from build123d import *

# Parameters (mm, degrees)
SKETCH2_W          = 125
SKETCH2_H          = 77.2
BASE_FLANGE1_DEPTH = 2
SKETCH2_3_W        = 3
SKETCH2_3_H        = 1.5
CUT_EXTRUDE1_DEPTH = 2
EDGE_FLANGE1_DEPTH = 50
SKETCH2_4_R        = 5
CUT_EXTRUDE2_DEPTH = 2
SKETCH12_R         = 5.5
CUT_EXTRUDE3_DEPTH = 2
FILLET1_R          = 3


# Sheet-metal steps are written as plain solids
with BuildPart() as part:
    # Sketch2 → Base-Flange1 (new body)
    with BuildSketch(Plane.XY):
        Rectangle(SKETCH2_W, SKETCH2_H)
    extrude(amount=-BASE_FLANGE1_DEPTH)

    # Sketch2<3> → Cut-Extrude1 (cut)
    with BuildSketch(Plane.XY):
        with Locations((-11, -37.85)):
            Rectangle(SKETCH2_3_W, SKETCH2_3_H)
    extrude(amount=-CUT_EXTRUDE1_DEPTH, mode=Mode.SUBTRACT)

    # Edge-Flange1 section (across the edge) → Edge-Flange1 (add)
    with BuildSketch(Plane(origin=(-62.5, -43.6, 0), x_dir=(0, 1, 0), z_dir=(1, 0, 0))):
        with BuildLine():
            Line((0, 0.7366), (0, 64.925))
            Line((0, 64.925), (2, 64.925))
            Line((2, 64.925), (2, 0.7366))
            ThreePointArc((2, 0.7366), (2.215745145, 0.215745145), (2.7366, 0))
            Line((2.7366, 0), (5, 0))
            Line((5, 0), (5, -2))
            Line((5, -2), (2.7366, -2))
            ThreePointArc((2.7366, -2), (0.801531583, -1.198468417), (0, 0.7366))
        make_face()
    extrude(amount=EDGE_FLANGE1_DEPTH)

    # Sketch2<4> → Cut-Extrude2 (cut)
    with BuildSketch(Plane.XY):
        with Locations((12.5, -11.4)):
            Circle(SKETCH2_4_R)
    extrude(amount=-CUT_EXTRUDE2_DEPTH, mode=Mode.SUBTRACT)

    # Sketch12 → Cut-Extrude3 (cut)
    with BuildSketch(Plane.XZ.offset(43.6)):
        with Locations(Location((-37.5, 39.925, 0), (0, 0, 270))):
            Circle(SKETCH12_R)
    extrude(amount=-CUT_EXTRUDE3_DEPTH, mode=Mode.SUBTRACT)

    # Fillet1
    fillet1_edges = [part.edges().sort_by_distance(p)[0] for p in [
        (-62.5, -42.6, 64.925),
        (-12.5, -42.6, 64.925),
        (62.5, 38.6, -1),
        (62.5, -38.6, -1),
        (-62.5, 38.6, -1),
    ]]
    fillet(fillet1_edges, radius=FILLET1_R)


solid = part.part
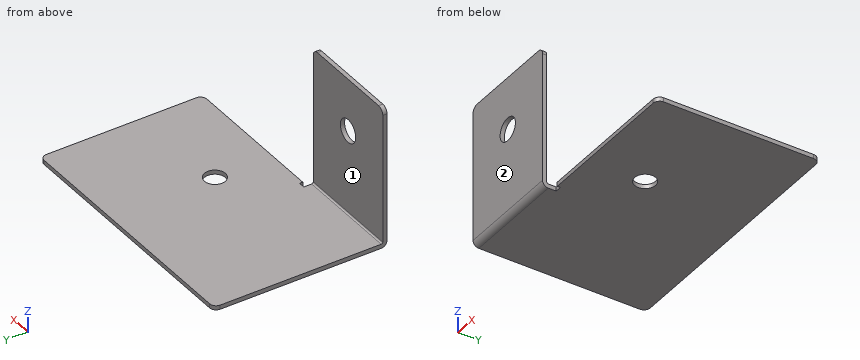
Check sheet for the modelled part. Datum: model origin and axes. Units: mm. Face numbers are marked on the shaded views. A direction names the side the tool comes from. Give positions to 0.01 mm unless a question says otherwise; leave off trailing zeros. Write each loop counter-clockwise with the first axis right and the second up, starting at its lowest first coordinate (ties: lowest second). Pieces come first, ordered by that corner, then holes. Notation, with made-up numbers: (25.25, 52.25) -> (34.25, 52.25) arc R11 cw to (34.25, 67.25) -> close; hole circle Ø7 at (6.5, 81.25). An arc over 180 degrees is marked (long way). Write item = value, one per line.
Item 1: Sectioned sample at D-D on z = 31.5. Record the boundary of the cut face in (x, y).
Output:
outline = (-62.5, -43.6) -> (-12.5, -43.6) -> (-12.5, -41.6) -> (-62.5, -41.6) -> close
Item 2: Gauge pin test, flat ends, axial feed: pin 1 (2 mm diameter, centred on x = 25, z = -0.5, fed in from -Y); pin 2 (1 mm diameter, centred on x = -11, z = -1.5, fed in from -Y); pin 3 (2 mm diameter, centred on x = -18, z = 19, fed in from +Y); pin 4 (11.5 mm diameter, centred on x = 12.5, y = -11.4, fed in from -Z). Record the tip position at first contact, or that the pin passes through.
Output:
pin_1 = -38.6
pin_2 = -37.1
pin_3 = -41.6
pin_4 = -2
Item 3: Sectioned sample at C-C on x = -37.5. Record the boundary of the cut face in (y, z) (3 decimals).
Output:
outline = (-43.6, 0.737) arc R2.737 ccw to (-40.863, -2) -> (38.6, -2) -> (38.6, 0) -> (-40.863, 0) arc R0.737 cw to (-41.6, 0.737) -> (-41.6, 34.425) -> (-43.6, 34.425) -> close; (-43.6, 45.425) -> (-41.6, 45.425) -> (-41.6, 64.925) -> (-43.6, 64.925) -> close
Item 4: Tool access check on the marked faces 1 and 2. Record the directions out of +Z, -Z, +X, -X, +Y, -Y that give a thin tool (end or side, any length) a straight path to the whole face; none if there is none.
Output:
face_1 = +Z, +X, -X, +Y
face_2 = +Z, -Z, +X, -X, -Y
Item 5: Sectioned sample at A-A on y = -11.4. Record the boundary of the cut face in (x, z), and give its area (3 significant figures).
Output:
outline = (-62.5, -2) -> (7.5, -2) -> (7.5, 0) -> (-62.5, 0) -> close; (17.5, -2) -> (62.5, -2) -> (62.5, 0) -> (17.5, 0) -> close
area = 230 mm^2
Item 6: Scan lines: probe 1 along Y at (x, z) = (12.5, -0.7); probe 2 along Z at (x, y) = (-54, -6); probe 3 along Y at (x, z) = (-26.5, 31). Record each from-to range of solid material in increasing order. Write a range as from..to.
Output:
probe_1 = -38.6..-16.4, -6.4..38.6
probe_2 = -2..0
probe_3 = -43.6..-41.6
Item 7: Sectioned sample at B-B on x = 12.5. Record the boundary of the cut face in (y, z), and give its area (3 significant figures).
Output:
outline = (-38.6, -2) -> (-16.4, -2) -> (-16.4, 0) -> (-38.6, 0) -> close; (-6.4, -2) -> (38.6, -2) -> (38.6, 0) -> (-6.4, 0) -> close
area = 134 mm^2
